```python
from build123d import *
from build123d.topology import SkipClean

# Parameters (mm, degrees)
SKETCH1_W                = 17.5
SKETCH1_H                = 3
SKETCH1_W_2              = 3
SKETCH1_H_2              = 17.5
BOSS_EXTRUDE1_DEPTH      = 45
FILLET1_R                = 2
CUT_EXTRUDE1_DEPTH       = 58.66714836
CUT_EXTRUDE1_DEPTH_BACK  = 58.66714836
SKETCH2_W                = 5
SKETCH2_H                = 30
CUT_EXTRUDE2_DEPTH       = 58.66714836
CUT_EXTRUDE2_DEPTH_BACK  = 58.66714836
SKETCH3_W                = 5
SKETCH3_H                = 30
CUT_EXTRUDE3_DEPTH       = 58.66714836
CUT_EXTRUDE3_DEPTH_BACK  = 58.66714836
SKETCH4_W                = 11
SKETCH4_H                = 23
CUT_EXTRUDE4_DEPTH       = 58.66714836
CUT_EXTRUDE4_DEPTH_BACK  = 58.66714836
SKETCH5_W                = 11
SKETCH5_H                = 23
SKETCH10_W               = 11
SKETCH10_H               = 4.5
CUT_EXTRUDE11_DEPTH      = 5
SKETCH6_W                = 11
SKETCH6_H                = 4.5
CUT_EXTRUDE12_DEPTH      = 4
SKETCH7_W                = 11
SKETCH7_H                = 4.5
CUT_EXTRUDE13_DEPTH      = 4
SKETCH11_W               = 11
SKETCH11_H               = 4.5
CUT_EXTRUDE14_DEPTH      = 3
CUT_EXTRUDE17_DEPTH      = 3
CUT_EXTRUDE17_DEPTH_BACK = 3
SKETCH13_W               = 11
SKETCH13_H               = 4.5


with BuildPart() as part:
    # Sketch1 → Boss-Extrude1 (new body)
    with BuildSketch(Plane(origin=(0, 0, 0), x_dir=(1, 0, 0), z_dir=(0, 1, 0))):
        with BuildLine():
            Line((-8.75, -23.951774465), (-8.75, -20.72890494))
            ThreePointArc((-8.75, -20.72890494), (-15.909902577, -15.909902577), (-20.72890494, -8.75))
            Line((-20.72890494, -8.75), (-23.951774465, -8.75))
            ThreePointArc((-23.951774465, -8.75), (-18.03122292, -18.03122292), (-8.75, -23.951774465))
        make_face()
        with BuildLine():
            Line((-23.951774465, -8.75), (-20.72890494, -8.75))
            ThreePointArc((-20.72890494, -8.75), (-22.5, 0), (-20.72890494, 8.75))
            Line((-20.72890494, 8.75), (-23.951774465, 8.75))
            ThreePointArc((-23.951774465, 8.75), (-25.10996066, 4.442957987), (-25.5, 2.1e-08))
            ThreePointArc((-25.5, 2.1e-08), (-25.109960663, -4.442957966), (-23.951774465, -8.75))
        make_face()
        with BuildLine():
            Line((-23.951774465, 8.75), (-20.72890494, 8.75))
            ThreePointArc((-20.72890494, 8.75), (-15.909902577, 15.909902577), (-8.75, 20.72890494))
            Line((-8.75, 20.72890494), (-8.75, 23.951774465))
            ThreePointArc((-8.75, 23.951774465), (-18.03122292, 18.03122292), (-23.951774465, 8.75))
        make_face()
        with BuildLine():
            Line((-8.75, 23.951774465), (-8.75, 20.72890494))
            ThreePointArc((-8.75, 20.72890494), (0, 22.5), (8.75, 20.72890494))
            Line((8.75, 20.72890494), (8.75, 23.951774465))
            ThreePointArc((8.75, 23.951774465), (4.442957973, 25.109960662), (-6e-09, 25.5))
            ThreePointArc((-6e-09, 25.5), (-4.442957979, 25.109960661), (-8.75, 23.951774465))
        make_face()
        with BuildLine():
            ThreePointArc((8.75, 20.72890494), (0, 22.5), (-8.75, 20.72890494))
            Line((-8.75, 20.72890494), (-8.75, 19.5))
            Line((-8.75, 19.5), (8.75, 19.5))
            Line((8.75, 19.5), (8.75, 20.72890494))
        make_face()
        with Locations((0, 18)):
            Rectangle(SKETCH1_W, SKETCH1_H)
        with Locations((-18, 0)):
            Rectangle(SKETCH1_W_2, SKETCH1_H_2)
        with BuildLine():
            ThreePointArc((-20.72890494, 8.75), (-22.5, 0), (-20.72890494, -8.75))
            Line((-20.72890494, -8.75), (-19.5, -8.75))
            Line((-19.5, -8.75), (-19.5, 8.75))
            Line((-19.5, 8.75), (-20.72890494, 8.75))
        make_face()
        with BuildLine():
            ThreePointArc((8.75, -20.72890494), (0, -22.5), (-8.75, -20.72890494))
            Line((-8.75, -20.72890494), (-8.75, -23.951774465))
            ThreePointArc((-8.75, -23.951774465), (-4.442957976, -25.109960662), (0, -25.5))
            ThreePointArc((0, -25.5), (4.442957976, -25.109960662), (8.75, -23.951774465))
            Line((8.75, -23.951774465), (8.75, -20.72890494))
        make_face()
        with BuildLine():
            Line((8.75, -19.500006), (-8.75, -19.500006))
            Line((-8.75, -19.500006), (-8.75, -20.72890494))
            ThreePointArc((-8.75, -20.72890494), (0, -22.5), (8.75, -20.72890494))
            Line((8.75, -20.72890494), (8.75, -19.500006))
        make_face()
        with Locations((0, -18.000006)):
            Rectangle(SKETCH1_W, SKETCH1_H)
        with BuildLine():
            ThreePointArc((20.72890494, -8.75), (15.909902577, -15.909902577), (8.75, -20.72890494))
            Line((8.75, -20.72890494), (8.75, -23.951774465))
            ThreePointArc((8.75, -23.951774465), (18.03122292, -18.03122292), (23.951774465, -8.75))
            Line((23.951774465, -8.75), (20.72890494, -8.75))
        make_face()
        with Locations((18, 0)):
            Rectangle(SKETCH1_W_2, SKETCH1_H_2)
        with BuildLine():
            Line((19.5, -8.75), (20.72890494, -8.75))
            ThreePointArc((20.72890494, -8.75), (22.052781697, -4.463722598), (22.5, 0))
            ThreePointArc((22.5, 0), (22.052781697, 4.463722598), (20.72890494, 8.75))
            Line((20.72890494, 8.75), (19.5, 8.75))
            Line((19.5, 8.75), (19.5, -8.75))
        make_face()
        with BuildLine():
            ThreePointArc((22.5, 0), (22.052781697, -4.463722598), (20.72890494, -8.75))
            Line((20.72890494, -8.75), (23.951774465, -8.75))
            ThreePointArc((23.951774465, -8.75), (25.109960662, -4.442957976), (25.5, 0))
            ThreePointArc((25.5, 0), (25.109960662, 4.442957976), (23.951774465, 8.75))
            Line((23.951774465, 8.75), (20.72890494, 8.75))
            ThreePointArc((20.72890494, 8.75), (22.052781697, 4.463722598), (22.5, 0))
        make_face()
        with BuildLine():
            ThreePointArc((8.75, 20.72890494), (15.909902577, 15.909902577), (20.72890494, 8.75))
            Line((20.72890494, 8.75), (23.951774465, 8.75))
            ThreePointArc((23.951774465, 8.75), (18.03122292, 18.03122292), (8.75, 23.951774465))
            Line((8.75, 23.951774465), (8.75, 20.72890494))
        make_face()
    extrude(amount=BOSS_EXTRUDE1_DEPTH)

    # Fillet1
    fillet1_edges = [part.edges().sort_by_distance(p)[0] for p in [
        (-20.72890494, 22.5, -8.75),
        (-20.72890494, 22.5, 8.75),
        (-8.75, 22.5, 20.72890494),
        (8.75, 22.5, 20.72890494),
        (20.72890494, 22.5, 8.75),
        (20.72890494, 22.5, -8.75),
        (8.75, 22.5, -20.72890494),
        (-8.75, 22.5, -20.72890494),
    ]]
    fillet(fillet1_edges, radius=FILLET1_R)

    # Sketch2 → Cut-Extrude1 (cut, two sides: drawn at the far end of the back side and taken through both)
    with BuildSketch(Plane(origin=(0, 0, 0), x_dir=(-0.7071067811865477, 0, -0.7071067811865475), z_dir=(0.7071067811865475, 0, -0.7071067811865477)).offset(-CUT_EXTRUDE1_DEPTH_BACK)):
        with Locations((0, 22.5)):
            Rectangle(SKETCH2_W, SKETCH2_H)
    extrude(amount=CUT_EXTRUDE1_DEPTH + CUT_EXTRUDE1_DEPTH_BACK, mode=Mode.SUBTRACT)

    # Sketch3 → Cut-Extrude2 (cut, two sides: drawn at the far end of the back side and taken through both)
    with BuildSketch(Plane(origin=(0, 0, 0), x_dir=(0.7071067811865476, 0, -0.7071067811865476), z_dir=(0.7071067811865476, 0, 0.7071067811865476)).offset(-CUT_EXTRUDE2_DEPTH_BACK)):
        with Locations((0, 22.5)):
            Rectangle(SKETCH3_W, SKETCH3_H)
    extrude(amount=CUT_EXTRUDE2_DEPTH + CUT_EXTRUDE2_DEPTH_BACK, mode=Mode.SUBTRACT)

    # Sketch4 → Cut-Extrude3 (cut, two sides: drawn at the far end of the back side and taken through both)
    with BuildSketch(Plane.XY.offset(-CUT_EXTRUDE3_DEPTH_BACK)):
        with Locations((0, 22.5)):
            Rectangle(SKETCH4_W, SKETCH4_H)
    extrude(amount=CUT_EXTRUDE3_DEPTH + CUT_EXTRUDE3_DEPTH_BACK, mode=Mode.SUBTRACT)

    # Sketch5 → Cut-Extrude4 (cut, two sides: drawn at the far end of the back side and taken through both)
    with BuildSketch(Plane(origin=(0, 0, 0), x_dir=(0, 0, -1), z_dir=(1, 0, 0)).offset(-CUT_EXTRUDE4_DEPTH_BACK)):
        with Locations((0, 22.5)):
            Rectangle(SKETCH5_W, SKETCH5_H)
    extrude(amount=CUT_EXTRUDE4_DEPTH + CUT_EXTRUDE4_DEPTH_BACK, mode=Mode.SUBTRACT)

    # Sketch10 → Cut-Extrude11 (cut)
    with BuildSketch(Plane(origin=(-16.5, 0, 0), x_dir=(0, 0, -1), z_dir=(1, 0, 0))):
        with Locations((0, 8.75)):
            Rectangle(SKETCH10_W, SKETCH10_H)
    extrude(amount=-CUT_EXTRUDE11_DEPTH, mode=Mode.SUBTRACT)

    # Sketch6 → Cut-Extrude12 (cut)
    with BuildSketch(Plane.ZY.offset(-16.5)):
        with Locations((0, 36.25)):
            Rectangle(SKETCH6_W, SKETCH6_H)
        with Locations((0, 8.75)):
            Rectangle(SKETCH6_W, SKETCH6_H)
    extrude(amount=-CUT_EXTRUDE12_DEPTH, mode=Mode.SUBTRACT)

    # Sketch7 → Cut-Extrude13 (cut)
    with BuildSketch(Plane(origin=(-16.5, 0, 0), x_dir=(0, 0, -1), z_dir=(1, 0, 0))):
        with Locations((0, 36.25)):
            Rectangle(SKETCH7_W, SKETCH7_H)
        with Locations((0, 8.75)):
            Rectangle(SKETCH7_W, SKETCH7_H)
    extrude(amount=-CUT_EXTRUDE13_DEPTH, mode=Mode.SUBTRACT)

    # Sketch11 → Cut-Extrude14 (cut)
    with SkipClean():  # the faces are left unmerged after this step: merging them gives an invalid solid
        with BuildSketch(Plane.XY.offset(25.500000054)):
            with Locations((0, 8.75)):
                Rectangle(SKETCH11_W, SKETCH11_H)
            with Locations((0, 36.25)):
                Rectangle(SKETCH11_W, SKETCH11_H)
        extrude(amount=-CUT_EXTRUDE14_DEPTH, mode=Mode.SUBTRACT)

    # Sketch13 → Cut-Extrude17 (cut, two sides: drawn at the far end of the back side and taken through both)
    with SkipClean():  # the faces are left unmerged after this step: merging them gives an invalid solid
        with BuildSketch(Plane.XY.offset(-25.500000054).offset(-CUT_EXTRUDE17_DEPTH_BACK)):
            with Locations((0, 36.25)):
                Rectangle(SKETCH13_W, SKETCH13_H)
            with Locations((0, 8.75)):
                Rectangle(SKETCH13_W, SKETCH13_H)
        extrude(amount=CUT_EXTRUDE17_DEPTH + CUT_EXTRUDE17_DEPTH_BACK, mode=Mode.SUBTRACT)


solid = part.part
```
Input: part model. Units: mm. Frame: model coordinates. A direction names the side the tool comes from. Give positions to 0.01 mm unless a question says otherwise; leave off trailing zeros. Loops run counter-clockwise (first coordinate to the right, second up) from the corner with the lowest first, then second, coordinate; pieces in that order, holes last.
1) Line query: L1, parallel to Z at x = 17.5, y = 38; L2, parallel to Z at x = 19, y = 22; L3, parallel to Z at x = -17, y = 29. Output: solid intervals per line, ascending.
A:
L1: z = -18.55 to -14.14, -8.75 to -5.5, 5.5 to 8.75, 14.14 to 18.55
L2: z = -15.46 to -12.05, -9.48 to -5.5, 5.5 to 9.48, 12.05 to 15.46
L3: z = -8.75 to -5.5, 5.5 to 8.75
2) Reachability of faces 1 (the flat face through (0, 36, -22.5)), 2 (the flat face through (-16.5, 22, -6)), 3 (the flat face through (-17, 37.5, 17)) from +Z, -Z, +X, -X, +Y, -Y: full face, straight path, thin tool, end or side. Return the list, or none.
A:
face 1: -Z
face 2: +Y, -Y
face 3: none
3) Section query B-B on x = 9.5. Return the cut outline in (y, z).
A:
outline: (0, -23.66) - (45, -23.66) - (45, -19.02) - (0, -19.02) - close; (0, 19.02) - (45, 19.02) - (45, 23.66) - (0, 23.66) - close
4) Section query C-C on z = -3. Return the cut outline in (x, y).
A:
outline: (-25.32, 0) - (-16.5, 0) - (-16.5, 6.5) - (-21.5, 6.5) - (-21.5, 11) - (-25.32, 11) - close; (-25.32, 34) - (-20.5, 34) - (-20.5, 38.5) - (-16.5, 38.5) - (-16.5, 45) - (-25.32, 45) - close; (16.5, 0) - (25.32, 0) - (25.32, 11) - (20.5, 11) - (20.5, 6.5) - (16.5, 6.5) - close; (16.5, 38.5) - (20.5, 38.5) - (20.5, 34) - (25.32, 34) - (25.32, 45) - (16.5, 45) - close
5) Contact query for flat-ended pins moving along their axis: pin 1 (6.5 mm diameter, centred on y = 30, z = -21, fed in from -X); pin 2 (1.5 mm diameter, centred on y = 20.5, z = -17, fed in from +X); pin 3 (9 mm diameter, centred on y = 19, z = 20, fed in from +X); pin 4 (3 mm diameter, centred on x = -2.5, y = 25.5, fed in from -Z). Output: stop coordinate, or through.
A:
pin 1: stops at x = -16.18
pin 2: stops at x = 14.21
pin 3: stops at x = 20.25
pin 4: passes through
6) Mould query, pull axis Z, two halves, no side actions, for faces 4 (the flat face through (-21, 22, 5.5)), 5 (the flat face through (-18.661, 22.29, -15.125)), 6 (the flat face through (0, 45, 17)). Classes: released by +Z, released by -Z, zero draft, split by the parting line, or undercut.
A:
face 4: undercut
face 5: released by -Z
face 6: zero draft
7) Section query A-A on z = -11. Return the cut outline in (x, y).
A:
outline: (-23.01, 0) - (-19.44, 0) - (-19.44, 45) - (-23.01, 45) - close; (19.44, 0) - (23.01, 0) - (23.01, 45) - (19.44, 45) - close
8) Section query D-D on y = 18. Count the separate pieces of the cut face and the enclosed holes in it, and give its area (3 significant figures).
A:
separate pieces: 8
enclosed holes: 0
area: 405 mm2
